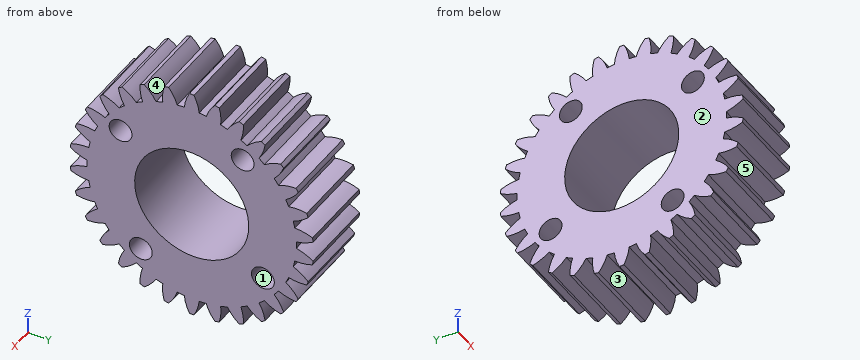
```python
from build123d import *

# Parameters (mm, degrees)
BASPROSKE_W        = 10
BASPROSKE_H        = 16
TOOTHCUT_DEPTH     = 25.738633754
TEETHCUTS_COUNT    = 30
TEETHCUTS_ANGLE    = 348
BORSKE_R           = 7.5
BORE_DEPTH         = 50.0000508
SKETCH1_R          = 1.5
CUT_EXTRUDE1_DEPTH = 25.700050474


with BuildPart() as part:
    # BasProSke → Base-Revolve (revolve)
    with BuildSketch(Plane(origin=(0, 0, 0), x_dir=(1, 0, 0), z_dir=(0, 1, 0)), mode=Mode.PRIVATE) as base_revolve_sk:
        with Locations((5, 8)):
            Rectangle(BASPROSKE_W, BASPROSKE_H)
    revolve(base_revolve_sk.sketch.rotate(Axis((-10, 0, 0), (1, 0, 0)), 180), axis=Axis((-10, 0, 0), (1, 0, 0)))

    # TooCutSke → ToothCut (cut, through all)
    with BuildSketch(Plane(origin=(0, 0, 0), x_dir=(0, 0, -1), z_dir=(1, 0, 0))):
        with BuildLine():
            ThreePointArc((0.466400716, 13.741086979), (0, 13.749), (-0.466400716, 13.741086979))
            ThreePointArc((-0.466400716, 13.741086979), (-0.819142092, 14.899954875), (-1.3974676, 15.964351834))
            ThreePointArc((-1.3974676, 15.964351834), (0, 16.0254), (1.3974676, 15.964351834))
            ThreePointArc((1.3974676, 15.964351834), (0.819142092, 14.899954875), (0.466400716, 13.741086979))
        make_face()
    toothcut = extrude(amount=TOOTHCUT_DEPTH, mode=Mode.SUBTRACT)

    # TeethCuts: ToothCut ×30 about axis
    teethcuts_axis = Axis((-10, 0, 0), (1, 0, 0))
    for i in range(1, TEETHCUTS_COUNT):
        add(toothcut.rotate(teethcuts_axis, i * TEETHCUTS_ANGLE / (TEETHCUTS_COUNT - 1)), mode=Mode.SUBTRACT)

    # BorSke → Bore (cut, symmetric)
    with BuildSketch(Plane(origin=(0, 0, 0), x_dir=(0, 0, -1), z_dir=(1, 0, 0))):
        with Locations(Location((0, 0, 0), (0, 0, 180))):
            Circle(BORSKE_R)
    extrude(amount=BORE_DEPTH, both=True, mode=Mode.SUBTRACT)

    # Sketch1 → Cut-Extrude1 (cut, through all)
    with BuildSketch(Plane.ZY):
        with Locations((6.689327089, -9.354298643)):
            Circle(SKETCH1_R)
        with Locations((9.354298643, 6.689327088)):
            Circle(SKETCH1_R)
        with Locations((-6.689327088, 9.354298643)):
            Circle(SKETCH1_R)
        with Locations((-9.354298643, -6.689327089)):
            Circle(SKETCH1_R)
    extrude(amount=-CUT_EXTRUDE1_DEPTH, mode=Mode.SUBTRACT)


solid = part.part
```
Here's how the part is built. I have some questions about the finished solid (model axes, mm). Face numbers are marked on the shaded views. A direction names the side the tool comes from. Give positions to 0.01 mm unless a question says otherwise; leave off trailing zeros. Write each loop counter-clockwise with the first axis right and the second up, starting at its lowest first coordinate (ties: lowest second). Pieces come first, ordered by that corner, then holes. Notation, with made-up numbers: M 89.5,3 L 143.5,3 A15 cw 143.5,22 Z; hole C 86.5,54 d4. An arc over 180 degrees is marked long. Put each result on its own line as item: value. Start each with the question number.
Item 1: Will these pins go through, and if not, where does the flat tip stop? pin 1 (1.8 mm diameter, centred on y = 6.69, z = 9.35, fed in from +X); pin 2 (6 mm diameter, centred on x = 6.5, z = -10, fed in from -Y); pin 3 (1 mm diameter, centred on x = 4, y = 9, fed in from +Z); pin 4 (1 mm diameter, centred on x = 5, y = 4.5, fed in from +Z).
Item 2: If we section it at B-B, the plane y = -1.5: Write out the boundary of the cut face in (x, z).
Item 3: If we section it at C-C, the plane x = 8.5: Count the separate pieces of the cut face and the enclosed holes in it, then the cut area to 3 significant figures.
Item 4: If we section it at A-A, the plane z = 0: Write out the boundary of the cut face in (x, y).
Item 5: On a 3-axis mill with a long thin cutter (end or side, diameter ignored), from which of +Z, -Z, +X, -X, +Y, -Y can I reach the whole of each face in a straight line? I mean the marked faces 3, 4 and 5. Say none if no direction works.
Item 6: Thinking about a two-plate mould opening in Y: for the marked faces 1 and 2, which applies, +Y half, -Y half, draft (parallel to the pull), parting line (faces both ways), or undercut?
Item 7: I need wall thicknesses on L1, parallel to Z at x = 6.75, y = 9; L2, parallel to Z at x = 9, y = 11.5; L3, parallel to Y at x = 2.5, z = -13.5. Which ranges of each line are inside material? Lowest first, please. Write a range as from..to.
Values:
1. pin 1: through
1. pin 2: y = -14
1. pin 3: z = 13.11
1. pin 4: z = 13.42
2. outline: M 0,-13.67 L 10,-13.67 L 10,-7.35 L 0,-7.35 Z; M 0,7.35 L 10,7.35 L 10,13.67 L 0,13.67 Z
3. separate pieces: 1
3. enclosed holes: 5
3. area: 486 mm²
4. outline: M 0,-13.75 L 10,-13.75 L 10,-7.5 L 0,-7.5 Z; M 0,7.5 L 10,7.5 L 10,13.75 L 0,13.75 Z
5. face 3: -Z, +X, -X
5. face 4: +Z, +X, -X
5. face 5: +X, -X
6. face 1: undercut
6. face 2: draft
7. L1: -13.03..-10.79, -10.39..-8.15, -5.23..10.39, 10.79..13.03
7. L2: -10.87..-9.3, -7.75..7.75, 9.3..10.87
7. L3: -6.76..-5.05, -3.83..3.83, 5.05..6.76
